Part model, mm, in its own coordinate system. A direction names the side the tool comes from. Give positions to 0.01 mm unless a question says otherwise; leave off trailing zeros. Write each loop counter-clockwise with the first axis right and the second up, starting at its lowest first coordinate (ties: lowest second). Pieces come first, ordered by that corner, then holes. Notation, with made-up numbers: M -26.75,84 L 4.25,84 A23 ccw 4.25,116 Z; hole C -2.75,30 d9. An arc over 180 degrees is marked long. Use CSV: the item, a comma, the result in double quotes. Start each with the question number.
1. Band-saw the part on C-C, the plane z = 36. List the corners of the cut face in (x, y), then the cut area to 3 significant figures.
2. Band-saw the part on B-B, the plane y = 0. List the corners of the cut face in (x, z), then the cut area to 3 significant figures.
3. Band-saw the part on A-A, the plane x = 0. List the corners of the cut face in (y, z).
4. Band-saw the part on D-D, the plane z = 7.5. List the corners of the cut face in (x, y), then the cut area to 3 significant figures.
5. Drop a flat-ended pin along its axis: pin 1 Ø1 at (y, z) = (1, 23.5) entering from -X. Give the stop position or say it passes through.
6. 3-axis set-ups, long thin cutter, end or side, ignore diameter. For faces 1 (the face through (-1.34, -0.06, 5.39)), 2 (the face through (0, 0, 35)): which of +Z, -Z, +X, -X, +Y, -Y reach the whole face in a straight line?
7. Mould opens along Y. For faces 3 (the face through (-4, 0, 22)), 4 (the face through (0, 0, 0)), 5 (the face through (-0.27, -1.22, 40.07)) say: pulls with the +Y half, pulls with the -Y half, needs draft (parallel to the pull), parting line crosses it, or undercut.
8. Drill centre lines: line 1 along Z through (x, y) = (0, 1.75); line 2 along X through (y, z) = (-0.25, 7.5); line 3 along Z through (x, y) = (1, 3.5). Where is each one in solid material? Low to high. Write a range as from..to.
Autodesk Inventor part; units mm, degrees
ref_plane "YZ Plane" through (0, 0, 0) normal (1, 0, 0) x (0, 1, 0)
ref_plane "XZ Plane" through (0, 0, 0) normal (0, 1, 0) x (-1, 0, 0)
ref_plane "XY Plane" through (0, 0, 0) normal (0, 0, 1) x (1, 0, 0)
sketch "Sketch1" plane through (0, 0, 0) normal (0, 0, 1) x (1, 0, 0)
  circle A0 centre (0, 0) radius 4
  dimension "d0" = 8
extrude "Extrusion1" add sketch "Sketch1" along normal blind 45
sketch "Sketch2" plane through (0, 0, 45) normal (0, 0, 1) x (1, 0, 0)
  circle A0 centre (0, 0) radius 1.25
  circle A1 centre (0, 0) radius 4
  dimension "d3" = 2.5
extrude "Extrusion2" cut sketch "Sketch2" against normal blind 10 contours A0
sketch "Sketch3" plane through (0, 0, 0) normal (0, 1, 0) x (-1, 0, 0)
  circle A0 centre (0, 7.5) radius 2.5
  line L0 (4, 0) -> (-4, 0)
  point P0 (0, 0)
  dimension "d6" = 5
  dimension "d7" = 7.5
extrude "Extrusion3" cut sketch "Sketch3" along normal mid plane 10
thread "Thread1"
fillet "Fillet1" radius 0.5 1 edges at (-4, 0, 45)
fillet "Fillet2" radius 0.5 1 edges at (-4, 0, 0)
properties part number "Drivescrew"
Output:
1,outline,"C 0,0 d8; hole C 0,0 d2.5"
1,area,"45.4 mm²"
2,outline,"M -4,0.5 A0.5 ccw -3.5,0 L 3.5,0 A0.5 ccw 4,0.5 L 4,44.5 A0.5 ccw 3.5,45 L 1.25,45 L 1.25,35 L -1.25,35 L -1.25,45 L -3.5,45 A0.5 ccw -4,44.5 Z; hole C 0,7.5 d5"
2,area,"315 mm²"
3,outline,"M -4,0.5 A0.5 ccw -3.5,0 L 3.5,0 A0.5 ccw 4,0.5 L 4,5 L -4,5 Z; M -4,10 L 4,10 L 4,44.5 A0.5 ccw 3.5,45 L 1.25,45 L 1.25,35 L -1.25,35 L -1.25,45 L -3.5,45 A0.5 ccw -4,44.5 Z"
4,outline,"M -2.5,-3.12 L -2.5,3.12 A4 ccw Z; M 2.5,-3.12 A4 ccw 2.5,3.12 Z"
4,area,"13.0 mm²"
5,pin 1,"stops at x = -3.97"
6,face 1,"+Y, -Y"
6,face 2,"+Z"
7,face 3,"parting line crosses it"
7,face 4,"needs draft"
7,face 5,"undercut"
8,line 1,"z = 0..5, 10..45"
8,line 2,"x = -3.99..-2.5, 2.5..3.99"
8,line 3,"z = 0.02..5.21, 9.79..44.98"
